Input: part model. Units: mm. Frame: model coordinates. Face numbers are marked on the shaded views. A direction names the side the tool comes from. Coordinates: 2 decimals unless noted, no trailing zeros. Loops run counter-clockwise (first coordinate to the right, second up) from the corner with the lowest first, then second, coordinate; pieces in that order, holes last. Notation, with made-up numbers: M 70,71 L 97,71 A20 ccw 97,96 Z; hole C -3,-9.5 d6. An arc over 180 degrees is marked long. Use a Markdown table: item, result. Add a question column.
1. Draft query along X for the marked faces 1, 2 and 3. Return one class per face: +X half, -X half, draft (parallel to the pull), parting line (faces both ways), or undercut.
2. Section A-A on x = 107. Output: boundary loops of the cut face in (y, z), then the cut area to 3 significant figures.
3. Pin query (flat end, axial travel): pin 1 (6.5 mm diameter, centred on x = 293.5, z = -46.5, fed in from +Y); pin 2 (5 mm diameter, centred on x = 273.5, z = -22, fed in from +Y); pin 3 (4.5 mm diameter, centred on x = 393.7, z = -65.09, fed in from +Y); pin 4 (10.5 mm diameter, centred on x = 273.5, y = 4.5, fed in from -Z). Return the tip coordinate at first contact, or that it passes through.
4. Set-up query: the marked faces 4, 5, 6, 7 and 8. Return all of +Z, -Z, +X, -X, +Y, -Y with unobstructed straight access to the full face (end or side cutting, diameter ignored); none if empty.
5. Section B-B on x = 61. Output: boundary loops of the cut face in (y, z).
6. Line query: L1, parallel to Y at x = 282.5, z = -20; L2, parallel to Z at x = 393, y = 40; L3, parallel to Y at x = 151, z = -23. Output: solid intervals per line, ascending. Write a range as [from, to].
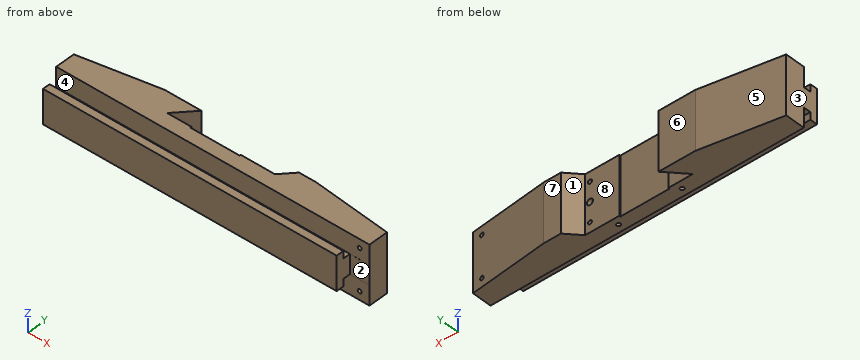
```python
from build123d import *

# Parameters (mm, degrees)
BOSS_EXTRUDE1_DEPTH         = 76.2
SKETCH4_W                   = 25.4
SKETCH4_H                   = 76.2
CUT_EXTRUDE2_DEPTH          = 19.1262
CUT_EXTRUDE9_DEPTH          = 419.232859396
F_1_4_20_TAPPED_HOLE1_D     = 5.1054
F_1_4_20_TAPPED_HOLE1_DEPTH = 12.7
F_1_4_20_TAPPED_HOLE1_TIP   = 1.533816902
F_3_8_16_TAPPED_HOLE1_D     = 7.9375
F_3_8_16_TAPPED_HOLE1_DEPTH = 25.4
F_3_8_16_TAPPED_HOLE1_TIP   = 2.384665582
F_1_4_20_TAPPED_HOLE2_D     = 5.1054
F_1_4_20_TAPPED_HOLE2_DEPTH = 11.1252
F_1_4_20_TAPPED_HOLE2_TIP   = 1.533816902
F_1_4_20_TAPPED_HOLE3_D     = 5.1054


with BuildPart() as part:
    # Sketch2 → Boss-Extrude1 (new body)
    with BuildSketch(Plane.XY):
        Polygon((0, 0), (406.4, 0), (406.4, 44.5262), (304.8, 55.6387), (282.423305624, 55.6387), (266.7, 38.1762), (222.25, 38.1762), (222.25, 36.5887), (158.75, 36.5887), (158.75, 38.1762), (127, 38.1762), (149.225, 62.859563142), (101.6, 62.859563142), (0, 44.5516), align=None)
    extrude(amount=-BOSS_EXTRUDE1_DEPTH)

    # Sketch4 → Cut-Extrude2 (cut)
    with BuildSketch(Plane(origin=(0, 0, 0), x_dir=(-1, 0, 0), z_dir=(0, -1, 0))):
        with Locations((-393.7, 38.1)):
            Rectangle(SKETCH4_W, SKETCH4_H)
    extrude(amount=-CUT_EXTRUDE2_DEPTH, mode=Mode.SUBTRACT)

    # Sketch7 → Cut-Extrude9 (cut, through all)
    with BuildSketch(Plane.ZY):
        Polygon((-76.2, 19.1516), (-76.2, -1.27), (-60.2869, -1.27), (-60.2869, 0.0254), (-60.2869, 9.5504), (-50.7619, 9.5504), (-50.7619, 19.1516), align=None)
        Polygon((-15.9131, 0.0254), (-15.9131, 9.5504), (-25.4381, 9.5504), (-25.4381, 19.1516), (0, 19.1516), (0, -1.27), (-15.9131, -1.27), align=None)
    extrude(amount=-CUT_EXTRUDE9_DEPTH, mode=Mode.SUBTRACT)

    # 1/4-20 Tapped Hole1
    with Locations(Plane(origin=(0, 0, -76.2), x_dir=(-1, 0, 0), z_dir=(0, 0, -1))):
        with Locations((-149.225, 28.6512), (-231.775, 28.6512)):
            Hole(F_1_4_20_TAPPED_HOLE1_D / 2, depth=F_1_4_20_TAPPED_HOLE1_DEPTH)
            with Locations((0, 0, -(F_1_4_20_TAPPED_HOLE1_DEPTH + F_1_4_20_TAPPED_HOLE1_TIP / 2))):  # 118° drill point
                Cone(0, F_1_4_20_TAPPED_HOLE1_D / 2, F_1_4_20_TAPPED_HOLE1_TIP, mode=Mode.SUBTRACT)

    # 3/8-16 Tapped Hole1
    with Locations(Plane(origin=(0, 38.1762, 0), x_dir=(1, 0, 0), z_dir=(0, 1, 0))):
        with Locations((260.35, 38.1)):
            Hole(F_3_8_16_TAPPED_HOLE1_D / 2, depth=F_3_8_16_TAPPED_HOLE1_DEPTH)
            with Locations((0, 0, -(F_3_8_16_TAPPED_HOLE1_DEPTH + F_3_8_16_TAPPED_HOLE1_TIP / 2))):  # 118° drill point
                Cone(0, F_3_8_16_TAPPED_HOLE1_D / 2, F_3_8_16_TAPPED_HOLE1_TIP, mode=Mode.SUBTRACT)

    # 1/4-20 Tapped Hole2
    with Locations(Plane(origin=(0, 38.1762, 0), x_dir=(1, 0, 0), z_dir=(0, 1, 0))):
        with Locations((260.35, 63.5), (260.35, 12.7)):
            Hole(F_1_4_20_TAPPED_HOLE2_D / 2, depth=F_1_4_20_TAPPED_HOLE2_DEPTH)
            with Locations((0, 0, -(F_1_4_20_TAPPED_HOLE2_DEPTH + F_1_4_20_TAPPED_HOLE2_TIP / 2))):  # 118° drill point
                Cone(0, F_1_4_20_TAPPED_HOLE2_D / 2, F_1_4_20_TAPPED_HOLE2_TIP, mode=Mode.SUBTRACT)

    # 1/4-20 Tapped Hole3 (through all)
    with Locations(Plane(origin=(0, 19.1516, 0), x_dir=(-1, 0, 0), z_dir=(0, -1, 0))):
        with Locations((-393.7, 11.1125), (-393.7, 65.0875)):
            Hole(F_1_4_20_TAPPED_HOLE3_D / 2)


solid = part.part
```
Answers below:
| question | item | result |
|---|---|---|
| 1 | face 1 | undercut |
| 1 | face 2 | draft |
| 1 | face 3 | -X half |
| 2 | outline | M 0,-60.29 L 9.55,-60.29 L 9.55,-50.76 L 19.15,-50.76 L 19.15,-76.2 L 62.86,-76.2 L 62.86,0 L 19.15,0 L 19.15,-25.44 L 9.55,-25.44 L 9.55,-15.91 L 0,-15.91 Z |
| 2 | area | 4,000 mm² |
| 3 | pin 1 | stops at y = 55.64 |
| 3 | pin 2 | stops at y = 48.5 |
| 3 | pin 3 | passes through |
| 3 | pin 4 | stops at z = -60.29 |
| 4 | face 4 | +Z, +X, -X |
| 4 | face 5 | +Z, -Z, -X, +Y |
| 4 | face 6 | +Z, -Z, +X, -X, +Y |
| 4 | face 7 | +Z, -Z, +X, +Y |
| 4 | face 8 | +Z, -Z, +Y |
| 5 | outline | M 0,-60.29 L 9.55,-60.29 L 9.55,-50.76 L 19.15,-50.76 L 19.15,-76.2 L 55.54,-76.2 L 55.54,0 L 19.15,0 L 19.15,-25.44 L 9.55,-25.44 L 9.55,-15.91 L 0,-15.91 Z |
| 6 | L1 | y = [0, 9.55], [19.15, 55.64] |
| 6 | L2 | z = [-76.2, -67.54], [-62.63, -13.57], [-8.66, 0] |
| 6 | L3 | y = [0, 9.55], [19.15, 38.18] |
